Build history of the part. All positions in model axes, mm. A direction names the side the tool comes from. Coordinates: 2 decimals unless noted, no trailing zeros. Order: outer loops, then holes, each group sorted by start corner. A loop starts at its lowest first (then second) coordinate and runs counter-clockwise, first axis right, second up. Notation, with made-up numbers: M -25,74.5 L 28,74.5 A14 ccw 28,82.5 Z; hole C 57,-8.75 d3. An arc over 180 degrees is marked long. Write item = value, one per line. Start each with the question number.
Q1. Band-saw the part on D-D on z = -72. Write the cut outline in (x, y), plus the area to 3 significant figures.
Q2. Band-saw the part on C-C on y = 105. Write the cut outline in (x, z), plus the area to 3 significant figures.
Q3. Pin check, flat tips, straight feed: P1, Ø4, axis at x = -17.5, z = -19, coming from the +Y side; P2, Ø8, axis at x = -38, y = -22, coming from the -Z side; P3, Ø0.8, axis at x = -100.5, z = -71, coming from the +Y side; P4, Ø21, axis at x = -64, z = -67.5, coming from the -Y side. Stop position of each tip, or through.
Q4. Drill centre lines: probe 1 along Z at (x, y) = (-49.5, 147); probe 2 along X at (y, z) = (43, -20); probe 3 along X at (y, z) = (49.5, -4.5). Where is each one in solid material? Low to high.
Q5. 3-axis set-ups, long thin cutter, end or side, ignore diameter. For faces 4 (the face through (-100, 64, -54)), 5 (the face through (-103, 29.907, -48)), 6 (the face through (-103, 45, -27.023)): which of +Z, -Z, +X, -X, +Y, -Y reach the whole face in a straight line?
Q6. Band-saw the part on B-B on z = -33. Write the cut outline in (x, y).
Q7. Pull direction Y, two halves, no side cores. Call faces 1 (the face through (-92.395, 64.623, -46.012)), 2 (the face through (-50.403, 5.548, -93.295)), 3 (the face through (-103, 60.366, -48)): released by +Y, released by -Y, zero draft, split by the parting line, or undercut.
Q8. Band-saw the part on A-A on x = -60. Write the cut outline in (y, z), plus the area to 3 significant figures.
```python
from build123d import *

# Parameters (mm, degrees)
SKETCH1_W           = 100
SKETCH1_H           = 100
BOSS_EXTRUDE1_DEPTH = 180
SKETCH2_R           = 34.257790197
BOSS_EXTRUDE2_DEPTH = 350
SKETCH3_W           = 152.006357392
SKETCH3_H           = 282.452416457
CUT_EXTRUDE2_DEPTH  = 400
CUT_EXTRUDE3_DEPTH  = 400
CUT_EXTRUDE4_DEPTH  = 400
CUT_EXTRUDE5_DEPTH  = 400
SKETCH7_W           = 160.159381639
SKETCH7_H           = 147.362276113
CUT_EXTRUDE6_DEPTH  = 400
SKETCH8_W           = 147.310744502
SKETCH8_H           = 162.038906966
CUT_EXTRUDE7_DEPTH  = 400
SKETCH9_R           = 31.847293423
CUT_EXTRUDE8_DEPTH  = 400
SKETCH10_W          = 140.220962397
SKETCH10_H          = 212.033531124
CUT_EXTRUDE9_DEPTH  = 400
SKETCH11_R          = 13.603137886
CUT_EXTRUDE11_DEPTH = 15
SKETCH12_R          = 12.495422516
BOSS_EXTRUDE3_DEPTH = 15
SKETCH13_R          = 1.594865099
BOSS_EXTRUDE4_DEPTH = 4
SKETCH14_W          = 100.74862993
SKETCH14_H          = 110.555003588
CUT_EXTRUDE13_DEPTH = 400
BOSS_EXTRUDE5_DEPTH = 1
SKETCH16_W          = 42.108585165
SKETCH16_H          = 30.458347221
BOSS_EXTRUDE6_DEPTH = 5


with BuildPart() as part:
    # Sketch1 → Boss-Extrude1 (new body)
    with BuildSketch(Plane(origin=(0, 0, 0), x_dir=(1, 0, 0), z_dir=(0, 1, 0))):
        with Locations((-50, 50)):
            Rectangle(SKETCH1_W, SKETCH1_H)
    extrude(amount=BOSS_EXTRUDE1_DEPTH)

    # Sketch2 → Boss-Extrude2 (add, symmetric)
    with BuildSketch(Plane(origin=(0, 180, 0), x_dir=(1, 0, 0), z_dir=(0, 1, 0))):
        with Locations(Location((-51.377291833, 49.076536384, 0), (0, 0, 270))):
            Circle(SKETCH2_R)
    extrude(amount=BOSS_EXTRUDE2_DEPTH, both=True)

    # Sketch3 → Cut-Extrude2 (cut)
    with BuildSketch(Plane(origin=(0, 0, 0), x_dir=(0, 0, -1), z_dir=(1, 0, 0))):
        with Locations((57.419900112, 502.274302507)):
            Rectangle(SKETCH3_W, SKETCH3_H)
    extrude(amount=-CUT_EXTRUDE2_DEPTH, mode=Mode.SUBTRACT)

    # Sketch4 → Cut-Extrude3 (cut)
    with BuildSketch(Plane(origin=(0, 0, 0), x_dir=(0, 0, -1), z_dir=(1, 0, 0))):
        Polygon((12.981970869, 0), (-8.994244796, 25.828096003), (-18.564506014, -15.259465835), align=None)
        Polygon((85.072517936, -1.448103984), (109.237639161, 19.113145112), (115.920034239, -3.267382694), align=None)
        Polygon((12.981970869, 180), (-8.994244796, 148.537596011), (-15.418178585, 193.219274892), align=None)
        Polygon((85.072517936, 181.854312784), (103.841225373, 159.795920888), (106.132549481, 198.647393934), align=None)
    extrude(amount=-CUT_EXTRUDE3_DEPTH, mode=Mode.SUBTRACT)

    # Sketch5 → Cut-Extrude4 (cut)
    with BuildSketch(Plane.XY):
        Polygon((-85.623287335, 0), (-106.370377984, 21.426392531), (-122.288861874, 3.209259887), (-93.526345261, -19.884701759), align=None)
        Polygon((-15.694988751, 0), (0, 15.257385304), (12.122677088, 15.257385304), (10.563067769, -19.884701759), align=None)
        Polygon((-87.166490339, 180.248071029), (-106.370377984, 151.29108453), (-117.705469457, 200.501115102), align=None)
        Polygon((-15.694988751, 180.248071029), (7.833767065, 153.279557508), (0, 193.941208308), align=None)
    extrude(amount=-CUT_EXTRUDE4_DEPTH, mode=Mode.SUBTRACT)

    # Sketch6 → Cut-Extrude5 (cut)
    with BuildSketch(Plane(origin=(0, 180, 0), x_dir=(1, 0, 0), z_dir=(0, 1, 0))):
        Polygon((-112.386997555, 28.400400964), (-64.261264503, -10.212759359), (-84.406366528, -15.51192827), (-124.649689542, -15.51192827), align=None)
        Polygon((-97.065537028, 135.861756084), (-119.37552445, 77.792688888), (-118.043343626, 64.347606737), (-66.428694172, 110.575168787), align=None)
        Polygon((-24.69640689, -21.815840769), (11.092108798, -8.97361337), (17.428316417, 32.393768119), (-38.531576846, -11.139157378), align=None)
        Polygon((-17.445484601, 140.804394854), (35.417473102, 107.262520599), (9.305452855, 72.996438725), (-31.724385352, 103.625272537), align=None)
    extrude(amount=-CUT_EXTRUDE5_DEPTH, mode=Mode.SUBTRACT)

    # Sketch7 → Cut-Extrude6 (cut)
    with BuildSketch(Plane.XY):
        with Locations((-66.123258915, -136.36252694)):
            Rectangle(SKETCH7_W, SKETCH7_H)
    extrude(amount=-CUT_EXTRUDE6_DEPTH, mode=Mode.SUBTRACT)

    # Sketch8 → Cut-Extrude7 (cut)
    with BuildSketch(Plane.XY):
        with Locations((-53.541153336, 332.448287589)):
            Rectangle(SKETCH8_W, SKETCH8_H)
    extrude(amount=-CUT_EXTRUDE7_DEPTH, mode=Mode.SUBTRACT)

    # Sketch9 → Cut-Extrude8 (cut)
    with BuildSketch(Plane(origin=(0, 251.428834106, 0), x_dir=(1, 0, 0), z_dir=(0, 1, 0))):
        with Locations(Location((-50.808993157, 49.032036374, 0), (0, 0, 270))):
            Circle(SKETCH9_R)
    extrude(amount=-CUT_EXTRUDE8_DEPTH, mode=Mode.SUBTRACT)

    # Sketch10 → Cut-Extrude9 (cut)
    with BuildSketch(Plane.ZY.offset(100)):
        with Locations((14.299084536, 180.100625535)):
            Rectangle(SKETCH10_W, SKETCH10_H)
    extrude(amount=-CUT_EXTRUDE9_DEPTH, mode=Mode.SUBTRACT)

    # Sketch11 → Cut-Extrude11 (cut)
    with BuildSketch(Plane.ZY.offset(100)):
        with Locations((-50.413251954, 76.264646142)):
            Circle(SKETCH11_R)
    extrude(amount=-CUT_EXTRUDE11_DEPTH, mode=Mode.SUBTRACT)

    # Sketch12 → Boss-Extrude3 (add)
    with BuildSketch(Plane.ZY.offset(85)):
        with Locations(Location((-50.658800768, 76.222522328, 0), (0, 0, 114.353089558))):
            Circle(SKETCH12_R)
    extrude(amount=BOSS_EXTRUDE3_DEPTH)

    # Sketch13 → Boss-Extrude4 (add)
    with BuildSketch(Plane(origin=(-85, 0, 0), x_dir=(0, 0, -1), z_dir=(1, 0, 0))):
        with Locations(Location((49.945205578, 75.944780088, 0), (0, 0, 180))):
            Circle(SKETCH13_R)
    extrude(amount=BOSS_EXTRUDE4_DEPTH)

    # Sketch14 → Cut-Extrude13 (cut)
    with BuildSketch(Plane.ZY.offset(100)):
        with Locations((-65.350029467, 250.603414818)):
            Rectangle(SKETCH14_W, SKETCH14_H)
    extrude(amount=-CUT_EXTRUDE13_DEPTH, mode=Mode.SUBTRACT)

    # Sketch15 → Boss-Extrude5 (add)
    with BuildSketch(Plane.ZY.offset(100)):
        Polygon((-18.461827727, 14.847435435), (-80.507743362, 14.847435435), (-80.507743362, 160.896793159), (-55.811396663, 160.896793159), (-55.811396663, 74.083859973), (-18.461827727, 74.083859973), align=None)
    extrude(amount=BOSS_EXTRUDE5_DEPTH)

    # Sketch16 → Boss-Extrude6 (add)
    with BuildSketch(Plane.ZY.offset(101)):
        with Locations((-48.07732297, 45.136437142)):
            Rectangle(SKETCH16_W, SKETCH16_H)
    extrude(amount=BOSS_EXTRUDE6_DEPTH)


solid = part.part
```
Recorded:
q1.outline = M -101,14.85 L -100,14.85 L -85.62,0 L -76.84,0 L -76.84,-62.68 L -72.87,-62.68 L -72.87,195.33 L -76.84,195.33 L -76.84,180 L -87.33,180 L -100,160.9 L -101,160.9 Z; M -28.75,-62.68 L -25.92,-62.68 L -25.92,0 L -15.69,0 L 0,15.26 L 0,162.26 L -15.48,180 L -25.92,180 L -25.92,195.33 L -28.75,195.33 Z
q1.area = 10,200 mm2
q2.outline = M -101,-80.51 L -100,-80.51 L -78.24,-100 L -26.87,-100 L 0,-79.94 L 0,-55.81 L -19.69,-55.81 A31.85 cw -81.93,-55.81 L -101,-55.81 Z
q2.area = 2,800 mm2
q3.P1 = 74.08
q3.P2 = -82.03
q3.P3 = 160.9
q3.P4 = -62.68
q4.probe_1 = -100 to -80.85
q4.probe_2 = -101 to -63.9, -37.72 to 0
q4.probe_3 = -82.6 to -18.43
q5.face_4 = none
q5.face_5 = +Z, -Z, -X, -Y
q5.face_6 = +Z, -X, +Y, -Y
q6.outline = M -106,29.91 L -101,29.91 L -101,14.85 L -100,14.85 L -85.62,0 L -81.63,0 L -81.63,-62.68 L -78.33,-62.68 L -78.33,74.08 L -101,74.08 L -101,60.37 L -106,60.37 Z; M -23.29,-62.68 L -21.13,-62.68 L -21.13,0 L -15.69,0 L 0,15.26 L 0,74.08 L -23.29,74.08 Z
q7.face_1 = undercut
q7.face_2 = released by -Y
q7.face_3 = released by +Y
q8.outline = M -62.68,-82.23 L 0,-82.23 L 0,-86.77 L 11.25,-100 L 164.31,-100 L 180,-86.65 L 180,-82.23 L 195.33,-82.23 L 195.33,-79.52 L -62.68,-79.52 Z; M -62.68,-18.54 L 74.08,-18.54 L 74.08,0 L 15.26,0 L 0,-12.98 L 0,-15.92 L -62.68,-15.92 Z
q8.area = 5,160 mm2
